```python
from build123d import *

# Parameters (mm, degrees)
F3_D = 45
F5_D = 3.1


with BuildPart() as f1:
    # F0 (on Right) → F1 (revolve)
    with BuildSketch(Plane.YZ):
        Polygon((0, -3), (0, 0), (-28, 0), (-28, -25), (-36, -25), (-36, -28), (-26.00142, -28), (-26.00142, -25), (-24.80142, -25), (-25, -3), align=None)
    revolve(axis=Axis((0, 0, -1.5), (0, 0, 1)))

    # F3 (through all)
    with Locations(Plane.XY):
        with Locations((0, 0)):
            Hole(F3_D / 2)

    # F5 (through all)
    with Locations(Plane.XY.offset(-25)):
        with Locations((-23.680949, -22.36131), (-31.911136, 0), (-24.321431, 20.12001), (0, 31.295169), (20.850252, 23.587119), (31.582344, 0), (21.738935, -24.314574), (0, -32.812748)):
            Hole(F5_D / 2)


solid = f1.part
```
The listing builds one solid part. Answer for the finished solid, in the listing's coordinates (mm). A direction names the side the tool comes from. Coordinates: 2 decimals unless noted, no trailing zeros. Loops run counter-clockwise (first coordinate to the right, second up) from the corner with the lowest first, then second, coordinate; pieces in that order, holes last. Notation, with made-up numbers: (-17.5, 27) -> (-8.5, 27) arc R13 ccw to (-8.5, 47) -> close; hole circle Ø4 at (12, 43). An arc over 180 degrees is marked (long way). Use one line per item in the form item = value. Start each with the question number.
Item 1: Consider L1, parallel to Z at x = -13, y = 25; L2, parallel to Y at x = 21, z = -20; L3, parallel to X at y = -2, z = -10. Determine where each line is inside the solid, lowest interval first. Write a range as [from, to].
Item 2: The part is cut by section A-A on x = 0. Count the separate pieces of the cut face and the enclosed holes in it, then the cut area to 3 significant figures.
Item 3: The part is cut by section C-C on z = -16.5. Determine the outline of the cut face in (x, y).
Item 4: The part is cut by section D-D on z = -21.75. Determine the outline of the cut face in (x, y), then the cut area to 3 significant figures.
Item 5: The mould has two halves that part along Y. Classify faces 1 (the face through (33.13, 0.07, -26.52)), 2 (the face through (-21, -19, -25)), 3 (the face through (35.694, 4.686, -26.521)), 4 (the face through (-10, -23, -25)): released by +Y, released by -Y, zero draft, split by the parting line, or undercut.
Item 6: A tool of negligible diameter and unlimited length cuts with its end or side. For faces 5 (the face through (-10.724, -25.865, -12.675)), 6 (the face through (-25.383, 5.637, -26.479)), 7 (the face through (-26.5, 0.2, -28)), 8 (the face through (7.48, -23.752, -13.846)), 9 (the face through (22.4, 23.66, -26.52)), from which of +Z, -Z, +X, -X, +Y, -Y can it reach the whole face along a straight path? Write none if from no direction.
Item 7: Flat-ended cylindrical pins translate along their axes: pin 1 Ø3 at (x, y) = (18, 28.5) entering from +Z; pin 2 Ø3 at (y, z) = (22, -18.5) entering from +X; pin 3 Ø1.5 at (y, z) = (19.5, -25) entering from -X. Find the tip coordinate at first contact, or state that the pin passes through.
Answer key:
q1.L1 = [-28, -25]
q1.L2 = [-18.52, -13.28], [13.28, 18.52]
q1.L3 = [-27.93, -24.86], [24.86, 27.93]
q2.separate_pieces = 4
q2.enclosed_holes = 0
q2.area = 211 mm2
q3.outline = circle Ø56 at (0, 0); hole circle Ø49.76 at (0, 0)
q4.outline = circle Ø56 at (0, 0); hole circle Ø49.66 at (0, 0)
q4.area = 526 mm2
q5.face_1 = undercut
q5.face_2 = zero draft
q5.face_3 = split by the parting line
q5.face_4 = undercut
q6.face_5 = +Z
q6.face_6 = -Z
q6.face_7 = -Z, +X, -X, +Y, -Y
q6.face_8 = none
q6.face_9 = +Z, -Z
q7.pin_1 = -25
q7.pin_2 = 19.07
q7.pin_3 = -30.73
